Job drawing, mm, ordinate dimensions from the low corner. One solid piece. A direction names the side the tool comes from. Give positions to 0.01 mm unless a question says otherwise; leave off trailing zeros. Order: outer loops, then holes, each group sorted by start corner. A loop starts at its lowest first (then second) coordinate and runs counter-clockwise, first axis right, second up. Notation, with made-up numbers: (49, 55.25) - (60, 55.25) arc R16 cw to (60, 59.25) - close; hole circle Ø7 at (2.5, 53.25). An arc over 180 degrees is marked (long way). Write each question's results on one line, items separated by ' | '. Start each with the question number.
1) Tool access for the marked faces 1, 2 and 3: list every direction of +Z, -Z, +X, -X, +Y, -Y with a clear straight run to the whole face (end or side of a thin tool).
2) Cut at C-C on y = 12.5. List the corners of the cut face in (x, z), plus the area to 3 significant figures.
3) Drop flat-ended pins along their axis: pin 1 Ø1.5 at (y, z) = (8.5, 37.5) entering from +X; pin 2 Ø10 at (x, z) = (116, 41) entering from -Y; pin 3 Ø24 at (x, y) = (31, 28.5) entering from +Z. Give the stop position or say it passes through.
4) Cut at D-D on z = 27.5. List the corners of the cut face in (x, y), plus the area to 3 significant figures.
5) Two-plate mould, pull along Y, no slides. Class the marked faces 4, 5 and 6: +Y half, -Y half, draft (parallel to the pull), parting line (faces both ways), or undercut.
6) Drill centre lines: line 1 along Y through (x, z) = (30, 56); line 2 along Z through (x, y) = (212, 31); line 3 along Z through (x, y) = (28, 55). Where is each one in solid material? Low to high. Write a range as from..to.
7) Cut at A-A on z = 62. List the corners of the cut face in (x, y), plus the area to 3 significant figures.
8) Cut at B-B on x = 30. List the corners of the cut face in (y, z), plus the area to 3 significant figures.
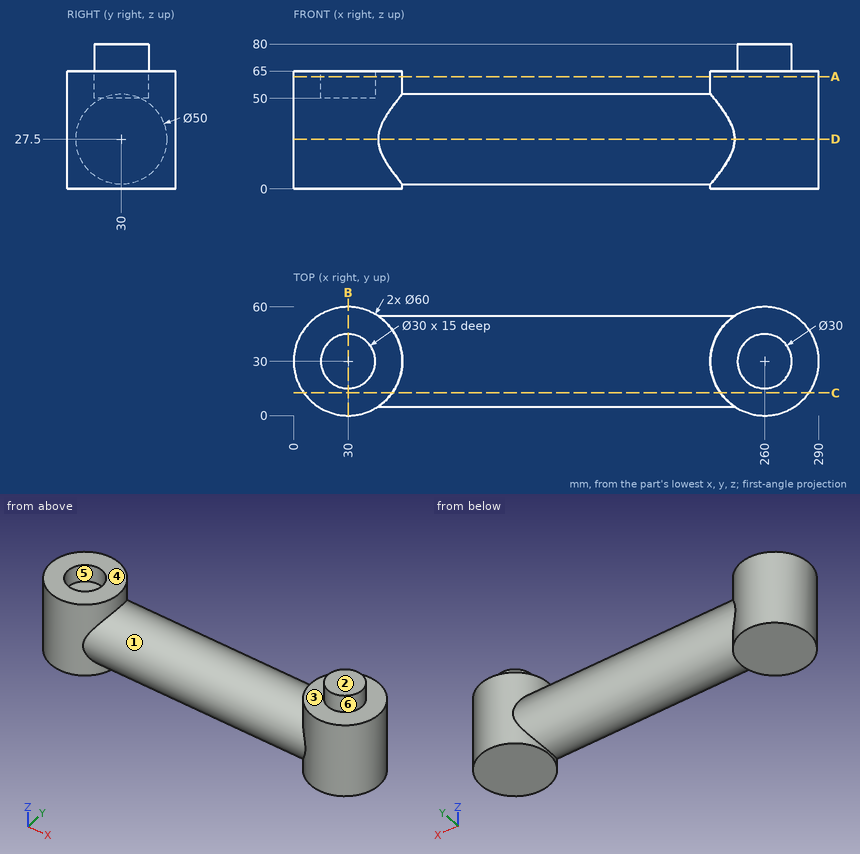
Results:
1) face 1: none | face 2: +Z, +X, -X, +Y, -Y | face 3: +Z
2) outline: (5.63, 0) - (54.37, 0) - (54.37, 9.65) - (235.63, 9.65) - (235.63, 0) - (284.37, 0) - (284.37, 65) - (235.63, 65) - (235.63, 45.35) - (54.37, 45.35) - (54.37, 65) - (5.63, 65) - close | area: 12,800 mm^2
3) pin 1: x = 281.67 | pin 2: y = 6.49 | pin 3: z = 50
4) outline: (46.58, 5) - (243.42, 5) arc R30 ccw (long way) to (243.42, 55) - (46.58, 55) arc R30 ccw (long way) to start | area: 14,600 mm^2
5) face 4: draft | face 5: undercut | face 6: parting line
6) line 1: 0..15, 45..60 | line 2: 2.52..52.48 | line 3: 0..65
7) outline: circle Ø60 at (30, 30); circle Ø60 at (260, 30); hole circle Ø30 at (30, 30) | area: 4,950 mm^2
8) outline: (0, 0) - (60, 0) - (60, 65) - (45, 65) - (45, 50) - (15, 50) - (15, 65) - (0, 65) - close | area: 3,450 mm^2
